Geometry check sheet. Reference: the model listing, model coordinates, mm. Face numbers are marked on the shaded views. Round coordinates to 2 decimals unless told otherwise and drop trailing zeros. Order: outer loops, then holes, each group sorted by start corner. A loop starts at its lowest first (then second) coordinate and runs counter-clockwise, first axis right, second up. Notation, with made-up numbers: (-31.5, -26.75) -> (2.5, -26.75) arc R8 cw to (2.5, -20.75) -> close; hole circle Ø4 at (33, 33). An arc over 180 degrees is marked (long way). Use a Markdown table: item, result. Add a question column.
Item 1: Sectioned sample at B-B, the plane y = -3. Record the cut outline in (x, z), and give its area (3 significant figures).
Item 2: Sectioned sample at C-C, the plane z = 7. Record the cut outline in (x, y).
Item 3: Sectioned sample at A-A, the plane x = 0. Record the cut outline in (y, z), and give its area (3 significant figures).
Item 4: Gauge pin test, flat ends, axial feed: pin 1 Ø2 at (x, z) = (-1.5, -6.5) entering from +Y; pin 2 Ø1 at (y, z) = (7.5, 16) entering from +X; pin 3 Ø10 at (x, y) = (-1, -1.5) entering from -Z. Record the tip position at first contact, or that the pin passes through.
Item 5: Material ranges on probe 1 along Y at (x, z) = (0, -36.7); probe 2 along Z at (x, y) = (-4.75, 0.5); probe 3 along Z at (x, y) = (-9.5, 3.75), recorded low to high. Write a range as [from, to].
Item 6: Mould release check, pull along Y, two halves, no side actions. Record for the marked faces 1, 2 and 3: pulls with the +Y half, pulls with the -Y half, needs draft (parallel to the pull), parting line crosses it, or undercut.
from build123d import *

# Parameters (mm, degrees)
BOSS_EXTRUDE1_DEPTH      = 35.5
BOSS_EXTRUDE1_DEPTH_BACK = 35.5
SKETCH1_R                = 10
CUT_EXTRUDE1_DEPTH       = 6
SKETCH3_R                = 4
BOSS_EXTRUDE2_DEPTH      = 7
SKETCH4_R                = 11.5
SKETCH4_R_2              = 8.5
BOSS_EXTRUDE3_DEPTH      = 2


with BuildPart() as part:
    # Sketch1 → Boss-Extrude1 (new, two sides: drawn at the far end of the back side and taken through both)
    with BuildSketch(Plane.XY.offset(-BOSS_EXTRUDE1_DEPTH_BACK)):
        Circle(SKETCH1_R)
    extrude(amount=BOSS_EXTRUDE1_DEPTH + BOSS_EXTRUDE1_DEPTH_BACK)

    # Sketch2 → Cut-Extrude1 (cut)
    with BuildSketch(Plane(origin=(0, 0, -35.5), x_dir=(-1, 0, 0), z_dir=(0, 0, -1))):
        Polygon((7.101408311, 0), (3.550704156, 6.15), (-3.550704156, 6.15), (-7.101408311, 0), (-3.550704156, -6.15), (3.550704156, -6.15), align=None)
    extrude(amount=-CUT_EXTRUDE1_DEPTH, mode=Mode.SUBTRACT)

    # Sketch3 → Boss-Extrude2 (add)
    with BuildSketch(Plane.XY.offset(35.5)):
        Circle(SKETCH3_R)
    extrude(amount=BOSS_EXTRUDE2_DEPTH)

    # Sketch4 → Boss-Extrude3 (add)
    with BuildSketch(Plane(origin=(0, 0, -35.5), x_dir=(-1, 0, 0), z_dir=(0, 0, -1))):
        Circle(SKETCH4_R)
        Circle(SKETCH4_R_2, mode=Mode.SUBTRACT)
    extrude(amount=BOSS_EXTRUDE3_DEPTH)


solid = part.part
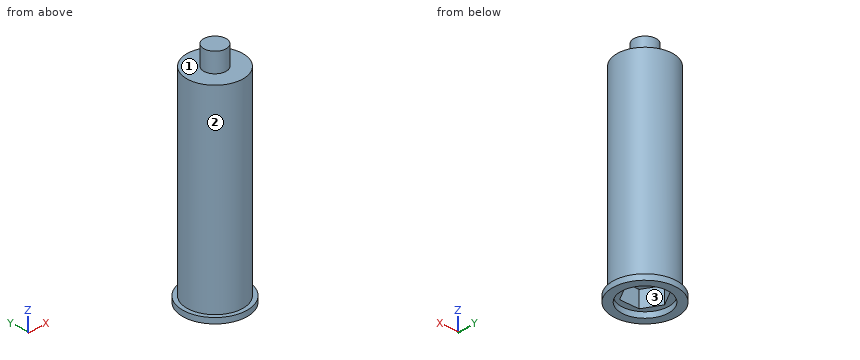
Found:
| question | item | result |
|---|---|---|
| 1 | outline | (-11.1, -37.5) -> (-7.95, -37.5) -> (-7.95, -35.5) -> (-5.37, -35.5) -> (-5.37, -29.5) -> (5.37, -29.5) -> (5.37, -35.5) -> (7.95, -35.5) -> (7.95, -37.5) -> (11.1, -37.5) -> (11.1, -35.5) -> (9.54, -35.5) -> (9.54, 35.5) -> (2.65, 35.5) -> (2.65, 42.5) -> (-2.65, 42.5) -> (-2.65, 35.5) -> (-9.54, 35.5) -> (-9.54, -35.5) -> (-11.1, -35.5) -> close |
| 1 | area | 1,340 mm2 |
| 2 | outline | circle Ø20 at (0, 0) |
| 3 | outline | (-11.5, -37.5) -> (-8.5, -37.5) -> (-8.5, -35.5) -> (-6.15, -35.5) -> (-6.15, -29.5) -> (6.15, -29.5) -> (6.15, -35.5) -> (8.5, -35.5) -> (8.5, -37.5) -> (11.5, -37.5) -> (11.5, -35.5) -> (10, -35.5) -> (10, 35.5) -> (4, 35.5) -> (4, 42.5) -> (-4, 42.5) -> (-4, 35.5) -> (-10, 35.5) -> (-10, -35.5) -> (-11.5, -35.5) -> close |
| 3 | area | 1,410 mm2 |
| 4 | pin 1 | stops at y = 9.99 |
| 4 | pin 2 | stops at x = 7.14 |
| 4 | pin 3 | stops at z = -35.5 |
| 5 | probe 1 | y = [-11.5, -8.5], [8.5, 11.5] |
| 5 | probe 2 | z = [-29.5, 35.5] |
| 5 | probe 3 | z = [-37.5, -35.5] |
| 6 | face 1 | needs draft |
| 6 | face 2 | parting line crosses it |
| 6 | face 3 | undercut |
